Here's how the part is built. I have some questions about the finished solid (model axes, mm). Coordinates: 2 decimals unless noted, no trailing zeros. Write each loop counter-clockwise with the first axis right and the second up, starting at its lowest first coordinate (ties: lowest second). Pieces come first, ordered by that corner, then holes.
Item 1: If we section it at A-A (z = 64): Please give me the cut outline in (x, y) (1 decimal), then the cut area to 3 significant figures.
Item 2: If we section it at B-B (y = 0.45): Count the separate pieces of the cut face and the enclosed holes in it, then the cut area to 3 significant figures.
Item 3: I'm going to push flat-ended pins straight in: pin 1 Ø5 at (x, z) = (245.5, -8) entering from -Y; pin 2 Ø4 at (x, z) = (204, 33.5) entering from -Y. Where does each tip first touch, or does it pass through?
Item 4: If I drill on line 1 (X direction, y = 0.25, z = -8.5) (3 decimals); line 2 (X direction, y = 0.5, z = 40.43) (3 decimals); line 3 (X direction, y = 0.1, z = 64) (3 decimals), over which ranges is the centre line in solid material (lowest first)?
Autodesk Inventor part; units mm, degrees
ref_plane "YZ Plane" through (0, 0, 0) normal (1, 0, 0) x (0, 1, 0)
ref_plane "XZ Plane" through (0, 0, 0) normal (0, 1, 0) x (-1, 0, 0)
ref_plane "XY Plane" through (0, 0, 0) normal (0, 0, 1) x (1, 0, 0)
sketch "Sketch1" plane through (0, 0, 0) normal (0, 1, 0) x (-1, 0, 0)
  line L0 (305.435, 114.3) -> (-305.435, 114.3)
  line L1 (-305.435, 114.3) -> (-305.435, -114.3)
  line L2 (-305.435, -114.3) -> (305.435, -114.3)
  line L3 (305.435, -114.3) -> (305.435, 114.3)
  line L4 (305.435, 114.3) -> (-305.435, -114.3) construction
  line L5 (-305.435, 114.3) -> (305.435, -114.3) construction
  point P0 (0, 0)
  dimension "d0" = 610.87
  dimension "d1" = 228.6
extrude "Extrusion1" add sketch "Sketch1" along normal blind 1.5875
sketch "Sketch2" plane through (0, 1.5875, 0) normal (0, 1, 0) x (1, 0, 0)
  circle A0 centre (204, 8) radius 34
  circle A1 centre (204, 49.5) radius 2.25
  circle A2 centre (174.6551, 37.3449) radius 2.25
  circle A3 centre (162.5, 8) radius 2.25
  circle A4 centre (174.6551, -21.3449) radius 2.25
  circle A5 centre (204, -33.5) radius 2.25
  circle A6 centre (233.3449, -21.3449) radius 2.25
  circle A7 centre (245.5, 8) radius 2.25
  circle A8 centre (233.3449, 37.3449) radius 2.25
  point P0 (0, 0)
  dimension "d4" = 68
  dimension "d6" = 4.5
  dimension "d7" = 41.5
  dimension "d10" = 360
  dimension "d15" = 204
  dimension "d16" = 8
extrude "Extrusion2" cut sketch "Sketch2" against normal blind 1.5875
sketch "Sketch3" plane through (0, 1.5875, 0) normal (0, 1, 0) x (1, 0, 0)
  circle A0 centre (4.6009, -64) radius 21
  circle A1 centre (204, 8) radius 34 construction
  circle A2 centre (204, 8) radius 106 construction
  circle A3 centre (-18.9691, -87.57) radius 2.55
  circle A4 centre (28.1709, -87.57) radius 2.55
  circle A5 centre (28.1709, -40.43) radius 2.55
  circle A6 centre (-18.9691, -40.43) radius 2.55
  line L0 (4.6009, -64) -> (204, 8) construction
  point P0 (0, 0)
  dimension "d17" = 42
  dimension "d18" = 212
  dimension "d20" = 72
  dimension "d21" = 5.1
  dimension "d22" = 23.57
  dimension "d23" = 23.57
  dimension "d26" = 360
  dimension "d30" = 212
extrude "Extrusion3" cut sketch "Sketch3" against normal through all
equation "\"d23\" = d22"
properties part number "ElectronicsBoxLid"
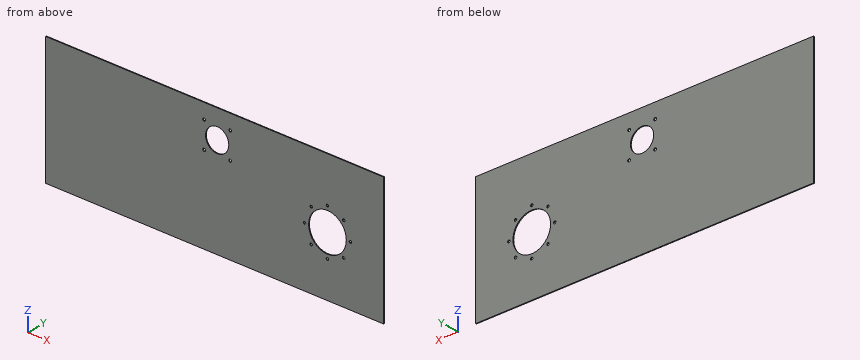
Answer list:
1. outline: (-305.4, 0) - (-16.4, 0) - (-16.4, 1.6) - (-305.4, 1.6) - close; (25.6, 0) - (305.4, 0) - (305.4, 1.6) - (25.6, 1.6) - close
1. area: 903 mm2
2. separate pieces: 1
2. enclosed holes: 14
2. area: 134,000 mm2
3. pin 1: stops at y = 0
3. pin 2: passes through
4. line 1: x = -305.435 to 160.306, 164.694 to 170.004, 237.996 to 243.306, 247.694 to 305.435
4. line 2: x = -305.435 to -21.519, -16.419 to 25.621, 30.721 to 305.435
4. line 3: x = -305.435 to -16.399, 25.601 to 305.435
